CAD build for the part. Positions are in the model's coordinates, mm. A direction names the side the tool comes from. Give positions to 0.01 mm unless a question says otherwise; leave off trailing zeros. Order: outer loops, then holes, each group sorted by start corner. A loop starts at its lowest first (then second) coordinate and runs counter-clockwise, first axis right, second up. Notation, with made-up numbers: (-20.5, 55) -> (3.5, 55) arc R17 ccw to (3.5, 80) -> close; hole circle Ø7 at (-28.5, 5). An arc over 180 degrees is marked (long way). Use one line per item in the form item = value. Start each with the question number.
1) Probe line 1 (X direction, y = 8.3, z = 0); line 2 (Y direction, x = -1.3, z = -0.8); line 3 (Z direction, x = 0.95, y = 10.5). List the from-to ranges inside material, lowest first.
2) Mould opens along Z. For faces 3 (the face through (0, 7.1, 0)), 4 (the face through (0, 0, 0)), 5 (the face through (1.109, 7.844, 1.958)), 6 (the face through (-0.27, 9.53, 1.22)) say: pulls with the +Z half, pulls with the -Z half, needs draft (parallel to the pull), parting line crosses it, or undercut.
3) Drop flat-ended pins along their axis: P1, Ø2, axis at x = 0, z = 0, coming from the +Y side; P2, Ø1, axis at y = 5.5, z = 2, coming from the +X side. Give the stop position or say it passes through.
4) Cut at C-C, the plane y = 3.5. Give the cut face in (x, z), and give its area (3 significant figures).
5) Cut at A-A, the plane y = 10.25. Give the cut face in (x, z), and give its area (3 significant figures).
6) Tool access for faces 1 (the face through (1.14, 7.84, -1.94)), 2 (the face through (1, 3.9, 1)): list every direction of +Z, -Z, +X, -X, +Y, -Y with a clear straight run to the whole face (end or side of a thin tool).
7) Cut at B-B, the plane y = 6. Give the cut face in (x, z), and give its area (3 significant figures).
from build123d import *

# Parameters (mm, degrees)
SKETCH1_R           = 1.25
BOSS_EXTRUDE1_DEPTH = 3.9
BOSS_EXTRUDE2_DEPTH = 8
SKETCH3_R           = 1.25
CUT_EXTRUDE2_DEPTH  = 4.8
SKETCH4_OUTSIDE_W   = 35.048
SKETCH4_OUTSIDE_H   = 35.744
SKETCH4_OUTSIDE_R   = 2.25
CUT_EXTRUDE3_DEPTH  = 12.9
CUT_EXTRUDE3_TAPER  = 45
SKETCH5_OUTSIDE_W   = 27.248
SKETCH5_OUTSIDE_H   = 27.944
SKETCH5_OUTSIDE_R   = 2.25
CUT_EXTRUDE6_DEPTH  = 9
CUT_EXTRUDE6_TAPER  = 45
CHAMFER2_SIZE       = 0.3
CHAMFER2_SIZE2      = 0.357526078


with BuildPart() as part:
    # Sketch1 → Boss-Extrude1 (new body)
    with BuildSketch(Plane(origin=(0, 0, 0), x_dir=(1, 0, 0), z_dir=(0, 1, 0))):
        Circle(SKETCH1_R)
    extrude(amount=BOSS_EXTRUDE1_DEPTH)

    # Sketch2 → Boss-Extrude2 (add)
    with BuildSketch(Plane(origin=(0, 3.9, 0), x_dir=(1, 0, 0), z_dir=(0, 1, 0))):
        Polygon((0, 2.598076211), (-2.25, 1.299038106), (-2.25, -1.299038106), (0, -2.598076211), (2.25, -1.299038106), (2.25, 1.299038106), align=None)
    extrude(amount=BOSS_EXTRUDE2_DEPTH)

    # Sketch3 → Cut-Extrude2 (cut)
    with BuildSketch(Plane(origin=(0, 11.9, 0), x_dir=(1, 0, 0), z_dir=(0, 1, 0))):
        Circle(SKETCH3_R)
    extrude(amount=-CUT_EXTRUDE2_DEPTH, mode=Mode.SUBTRACT)

    # Sketch4 outside → Cut-Extrude3 (cut, through all)
    with BuildSketch(Plane(origin=(0, 11.9, 0), x_dir=(1, 0, 0), z_dir=(0, 1, 0))):
        Rectangle(SKETCH4_OUTSIDE_W, SKETCH4_OUTSIDE_H)
        Circle(SKETCH4_OUTSIDE_R, mode=Mode.SUBTRACT)
    extrude(amount=-CUT_EXTRUDE3_DEPTH, taper=CUT_EXTRUDE3_TAPER, mode=Mode.SUBTRACT)

    # Sketch5 outside → Cut-Extrude6 (cut, through all)
    with BuildSketch(Plane.XZ.offset(-3.9)):
        Rectangle(SKETCH5_OUTSIDE_W, SKETCH5_OUTSIDE_H)
        Circle(SKETCH5_OUTSIDE_R, mode=Mode.SUBTRACT)
    extrude(amount=-CUT_EXTRUDE6_DEPTH, taper=CUT_EXTRUDE6_TAPER, mode=Mode.SUBTRACT)

    # Chamfer2
    chamfer2_edges = [part.edges().sort_by_distance(p)[0] for p in [
        (-1.25, 0, 0),
    ]]
    chamfer2_side = [part.faces().sort_by_distance(p)[0] for p in [
        (0, 0, 0),
    ]]
    chamfer(chamfer2_edges, length=CHAMFER2_SIZE, length2=CHAMFER2_SIZE2, reference=chamfer2_side[0])


solid = part.part
Result:
q1.line_1 = -2.25 to -1.25, 1.25 to 2.25
q1.line_2 = 3.9 to 11.9
q1.line_3 = -2.05 to -0.81, 0.81 to 2.05
q2.face_3 = undercut
q2.face_4 = needs draft
q2.face_5 = pulls with the +Z half
q2.face_6 = undercut
q3.P1 = 7.1
q3.P2 = 1.9
q4.outline = circle Ø2.5 at (0, 0)
q4.area = 4.91 mm²
q5.outline = (-2.25, -1.3) -> (0, -2.6) -> (2.25, -1.3) -> (2.25, 1.3) -> (0, 2.6) -> (-2.25, 1.3) -> close; hole circle Ø2.5 at (0, 0)
q5.area = 12.6 mm²
q6.face_1 = -Z, +X, +Y, -Y
q6.face_2 = -Y
q7.outline = (-2.25, -1.3) -> (0, -2.6) -> (2.25, -1.3) -> (2.25, 1.3) -> (0, 2.6) -> (-2.25, 1.3) -> close
q7.area = 17.5 mm²
